Read the model definition and answer for the solid it produces. Units are mm, in the model's axes. Face numbers are marked on the shaded views. A direction names the side the tool comes from. Give positions to 0.01 mm unless a question says otherwise; leave off trailing zeros. Order: outer loops, then holes, each group sorted by start corner. A loop starts at its lowest first (then second) coordinate and runs counter-clockwise, first axis right, second up. Notation, with made-up numbers: (17, -21) - (40, -21) arc R14 cw to (40, -15) - close; hole circle Ø9 at (-28.75, -7). An arc over 180 degrees is marked (long way). Use a Markdown table: item, result. Add a question column.
1. For a pull along X with two mould halves and no side action, classify the marked faces 1, 2 and 3 as released by +X, released by -X, zero draft, split by the parting line, or undercut.
2. A cutting plane is placed at C-C on x = -12. Determine the outline of the cut face in (y, z).
3. Which of the six approach directions +Z, -Z, +X, -X, +Y, -Y give full straight-line access (tool end or side, diameter ignored) to the marked faces 4, 5 and 6?
4. Flat-ended cylindrical pins translate along their axes: P1, Ø1.6, axis at x = -45, y = 8, coming from the -Z side; P2, Ø1.6, axis at x = 15.5, y = 0.5, coming from the +Z side; P3, Ø1.2, axis at x = 44.5, z = 42.5, coming from the -Y side. Find the tip coordinate at first contact, or state that the pin passes through.
5. A cutting plane is placed at B-B on z = 41. Determine the outline of the cut face in (x, y).
6. A cutting plane is placed at A-A on y = 4.5. Determine the outline of the cut face in (x, z), and give its area (3 significant figures).
7. Consider L1, parallel to X at y = 9, z = 40.5; L2, parallel to X at y = 0.75, z = 43.75; L3, parallel to Y at x = 32, z = 41.75. Determine where each line is inside the solid, lowest interval first.
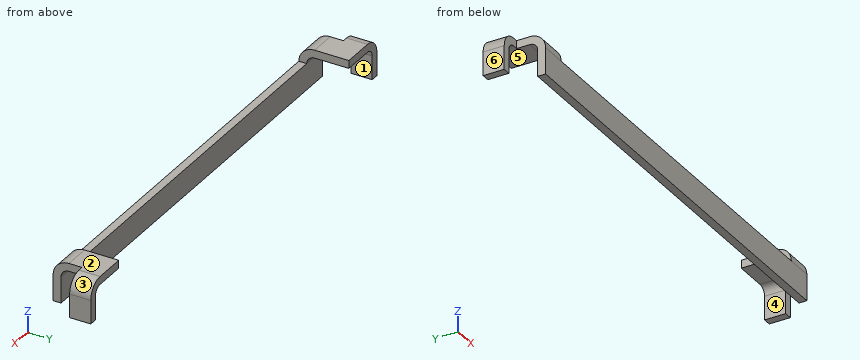
```python
from build123d import *

# Parameters (mm, degrees)
BOSS_EXTRUDE1_DEPTH        = 1.5
SKETCH3_W                  = 5
SKETCH3_H                  = 1.5
BOSS_EXTRUDE2_DEPTH        = 8
BOSS_EXTRUDE3_DEPTH        = 6
BOSS_EXTRUDE3_DEPTH_BACK   = 1.5
SKETCH4_W                  = 1.5
SKETCH4_H                  = 4
BOSS_EXTRUDE3_2_DEPTH      = 6
BOSS_EXTRUDE3_2_DEPTH_BACK = 1.5
SKETCH5_W                  = 2.5
SKETCH5_H                  = 1.5
BOSS_EXTRUDE4_DEPTH        = 4
CONVERT_SOLID2_START       = 5.5
CONVERT_SOLID2_DEPTH       = 4
CONVERT_SOLID2_START_2     = -42
CONVERT_SOLID2_2_DEPTH     = 5
CONVERT_SOLID2_START_3     = 37
CONVERT_SOLID2_3_DEPTH     = 5
CONVERT_SOLID2_4_DEPTH     = 4
CONVERT_SOLID2_5_DEPTH     = 84
CUT_EXTRUDE1_DEPTH         = 10


# Read off the part's stored shape, not the designer's step: Convert-Solid2
with BuildPart() as part:
    # Sketch1 → Boss-Extrude1 (new body)
    with BuildSketch(Plane(origin=(0, 0, 0), x_dir=(1, 0, 0), z_dir=(0, 1, 0))):
        Polygon((-42, -45.5), (-42, -42.5), (-45, -42.5), (-45, 42.5), (45, 42.5), (45, -42.5), (42, -42.5), (42, -45.5), (37, -45.5), (37, -42.5), (-37, -42.5), (-37, -45.5), align=None)
    extrude(amount=BOSS_EXTRUDE1_DEPTH)

    # Sketch3 → Boss-Extrude2 (add)
    with BuildSketch(Plane(origin=(0, 1.5, 0), x_dir=(1, 0, 0), z_dir=(0, 1, 0))):
        with Locations((-39.5, -44.75)):
            Rectangle(SKETCH3_W, SKETCH3_H)
        with Locations((39.5, -44.75)):
            Rectangle(SKETCH3_W, SKETCH3_H)
    extrude(amount=BOSS_EXTRUDE2_DEPTH)



with BuildPart() as body_2:
    # Sketch4 → Boss-Extrude3 (new, two sides: drawn at the far end of the back side and taken through both)
    with BuildSketch(Plane(origin=(0, 0, 44), x_dir=(-1, 0, 0), z_dir=(0, 0, -1)).offset(-BOSS_EXTRUDE3_DEPTH_BACK)):
        with Locations((45.25, 7.5)):
            Rectangle(SKETCH4_W, SKETCH4_H)
    extrude(amount=BOSS_EXTRUDE3_DEPTH + BOSS_EXTRUDE3_DEPTH_BACK)


with BuildPart() as body_3:
    # Sketch4 → Boss-Extrude3 2 (new, two sides: drawn at the far end of the back side and taken through both)
    with BuildSketch(Plane(origin=(0, 0, 44), x_dir=(-1, 0, 0), z_dir=(0, 0, -1)).offset(-BOSS_EXTRUDE3_2_DEPTH_BACK)):
        with Locations((-45.25, 7.5)):
            Rectangle(SKETCH4_W, SKETCH4_H)
    extrude(amount=BOSS_EXTRUDE3_2_DEPTH + BOSS_EXTRUDE3_2_DEPTH_BACK)


with BuildPart() as part_1:
    add(part.part)

    add(body_2.part)  # Boss-Extrude4 merges body 2

    add(body_3.part)  # Boss-Extrude4 merges body 3
    # Sketch5 → Boss-Extrude4 (add)
    with BuildSketch(Plane(origin=(0, 9.5, 0), x_dir=(1, 0, 0), z_dir=(0, 1, 0))):
        with Locations((-43.25, -44.75)):
            Rectangle(SKETCH5_W, SKETCH5_H)
        with Locations((43.25, -44.75)):
            Rectangle(SKETCH5_W, SKETCH5_H)
    extrude(amount=-BOSS_EXTRUDE4_DEPTH)

    # Convert-Solid2 outline → Convert-Solid2 (add)
    with BuildSketch(Plane(origin=(0, 0, 0), x_dir=(1, 0, 0), z_dir=(0, 1, 0)).offset(CONVERT_SOLID2_START)):
        with BuildLine():
            ThreePointArc((44.5, -42.5), (44.060660172, -43.560660172), (43, -44))
            Line((43, -44), (44.5, -44))
            Line((44.5, -44), (44.5, -42.5))
        make_face()
        with BuildLine():
            ThreePointArc((-43, -44), (-44.060660172, -43.560660172), (-44.5, -42.5))
            Line((-44.5, -42.5), (-44.5, -44))
            Line((-44.5, -44), (-43, -44))
        make_face()
    extrude(amount=CONVERT_SOLID2_DEPTH)

    # Convert-Solid2 2 outline → Convert-Solid2 2 (add)
    with BuildSketch(Plane.YZ.offset(CONVERT_SOLID2_START_2)):
        with BuildLine():
            ThreePointArc((1.5, 42.5), (1.939339828, 43.560660172), (3, 44))
            Line((3, 44), (1.5, 44))
            Line((1.5, 44), (1.5, 42.5))
        make_face()
    extrude(amount=CONVERT_SOLID2_2_DEPTH)

    # Convert-Solid2 3 outline → Convert-Solid2 3 (add)
    with BuildSketch(Plane.YZ.offset(CONVERT_SOLID2_START_3)):
        with BuildLine():
            ThreePointArc((1.5, 42.5), (1.939339828, 43.560660172), (3, 44))
            Line((3, 44), (1.5, 44))
            Line((1.5, 44), (1.5, 42.5))
        make_face()
    extrude(amount=CONVERT_SOLID2_3_DEPTH)

    # Convert-Solid2 4 outline → Convert-Solid2 4 (cut)
    with BuildSketch(Plane(origin=(0, 0, 0), x_dir=(1, 0, 0), z_dir=(0, 1, 0)).offset(CONVERT_SOLID2_START)):
        with BuildLine():
            ThreePointArc((46, -42.5), (45.121320344, -44.621320344), (43, -45.5))
            Line((43, -45.5), (46, -45.5))
            Line((46, -45.5), (46, -42.5))
        make_face()
        with BuildLine():
            ThreePointArc((-43, -45.5), (-45.121320344, -44.621320344), (-46, -42.5))
            Line((-46, -42.5), (-46, -45.5))
            Line((-46, -45.5), (-43, -45.5))
        make_face()
    extrude(amount=CONVERT_SOLID2_4_DEPTH, mode=Mode.SUBTRACT)

    # Convert-Solid2 5 outline → Convert-Solid2 5 (cut)
    with BuildSketch(Plane.YZ.offset(CONVERT_SOLID2_START_2)):
        with BuildLine():
            ThreePointArc((0, 42.5), (0.878679656, 44.621320344), (3, 45.5))
            Line((3, 45.5), (0, 45.5))
            Line((0, 45.5), (0, 42.5))
        make_face()
    extrude(amount=CONVERT_SOLID2_5_DEPTH, mode=Mode.SUBTRACT)

    # Sketch6 → Cut-Extrude1 (cut)
    with BuildSketch(Plane(origin=(0, 1.5, 0), x_dir=(1, 0, 0), z_dir=(0, 1, 0))):
        Polygon((-45, 42.5), (45, 42.5), (45, -37.5), (45, -42.5), (42, -42.5), (42, -37.5), (-42, -37.5), (-42, -42.5), (-45, -42.5), (-45, -37.5), align=None)
    extrude(amount=-CUT_EXTRUDE1_DEPTH, mode=Mode.SUBTRACT)


solid = part_1.part
```
Output values:
| question | item | result |
|---|---|---|
| 1 | face 1 | undercut |
| 1 | face 2 | zero draft |
| 1 | face 3 | released by +X |
| 2 | outline | (0, 37.5) - (1.5, 37.5) - (1.5, 42.5) - (0, 42.5) - close |
| 3 | face 4 | -Z, +Y, -Y |
| 3 | face 5 | -Z, +Y |
| 3 | face 6 | +Z, -Z, -X, +Y, -Y |
| 4 | P1 | z = 38 |
| 4 | P2 | z = 42.5 |
| 4 | P3 | y = 5.5 |
| 5 | outline | (-46, 5.5) - (-44.5, 5.5) - (-44.5, 9.5) - (-46, 9.5) - close; (-42, 0) - (42, 0) - (42, 1.5) - (-42, 1.5) - close; (44.5, 5.5) - (46, 5.5) - (46, 9.5) - (44.5, 9.5) - close |
| 6 | outline | (-42, 44) - (-37, 44) - (-37, 45.5) - (-42, 45.5) - close; (37, 44) - (42, 44) - (42, 45.5) - (37, 45.5) - close |
| 6 | area | 15.0 mm² |
| 7 | L1 | -46 to -44.5, 44.5 to 46 |
| 7 | L2 | -42 to -37, 37 to 42 |
| 7 | L3 | 0 to 1.5 |
